Geometry: final body of the model. Coordinates: model frame, mm. Give positions to 0.01 mm unless a question says otherwise; leave off trailing zeros. Write each loop counter-clockwise with the first axis right and the second up, starting at its lowest first coordinate (ties: lowest second). Pieces come first, ordered by that corner, then holes.
Q1. Section B-B (x = -337). Return the cut outline in (y, z) (3 decimals), plus the area to 3 significant figures.
Q2. Section A-A (z = 12.75). Return the cut outline in (x, y), plus the area to 3 significant figures.
Q3. Line query: line 1 (Y direction, x = -16, z = 18); line 2 (X direction, y = 50, z = 16.5); line 3 (X direction, y = 34, z = 8.5). Output: solid intervals per line, ascending.
Q4. Pin query (flat end, axial travel): pin 1 Ø3 at (y, z) = (65, 12) entering from +X; pin 2 Ø1 at (y, z) = (27, 12) entering from -X; pin 3 Ø1 at (y, z) = (34.5, 13) entering from -X. Return the tip coordinate at first contact, or that it passes through.
Q5. Section C-C (y = 15.5). Return the cut outline in (x, z), plus the area to 3 significant figures.
Autodesk Inventor part; units mm, degrees
ref_plane "YZ Plane" through (0, 0, 0) normal (1, 0, 0) x (0, 1, 0)
ref_plane "XZ Plane" through (0, 0, 0) normal (0, 1, 0) x (-1, 0, 0)
ref_plane "XY Plane" through (0, 0, 0) normal (0, 0, 1) x (1, 0, 0)
sketch "Sketch2" plane through (0, 0, 0) normal (0, 0, 1) x (1, 0, 0)
  line L0 (-410.0497, 90.9112) -> (409.1003, 90.9112)
  line L1 (409.1003, 90.9112) -> (409.1003, -10.6888)
  line L2 (409.1003, -10.6888) -> (-410.0497, -10.6888)
  line L3 (-410.0497, -10.6888) -> (-410.0497, 90.9112)
  point P0 (0, 0)
  dimension "d0" = 819.15
  dimension "d1" = 101.6
extrude "Board" add sketch "Sketch2" along normal blind 19.05
sketch "Sketch10" plane through (0, 0, 19.05) normal (0, 0, 1) x (1, 0, 0)
  line L0 (409.1003, -10.6888) -> (409.1003, 90.9112)
  line L1 (409.1003, 81.3862) -> (-410.0497, 81.3862)
  line L2 (-410.0497, 81.3862) -> (-410.0497, 71.8612)
  line L3 (-410.0497, 71.8612) -> (409.1003, 71.8612)
  line L4 (409.1003, 71.8612) -> (409.1003, 81.3862)
  line L5 (-410.0497, 90.9112) -> (-410.0497, -10.6888)
  line L6 (409.1003, 90.9112) -> (-410.0497, 90.9112)
  point P0 (0, 0)
  dimension "d22" = 9.525
  dimension "d23" = 9.525
sketch "Sketch8" plane through (-410.0497, -10.6888, 0) normal (0, -1, 0) x (1, 0, 0)
  line L0 (819.15, 19.05) -> (0, 19.05)
  line L1 (0, 0) -> (0, 19.05)
  line L2 (0, 19.05) -> (0, 0)
  line L3 (0, 0) -> (19.05, 19.05)
  line L4 (19.05, 19.05) -> (0, 19.05)
  line L5 (819.15, 0) -> (819.15, 19.05)
  line L6 (819.15, 19.05) -> (819.15, 0)
  line L7 (819.15, 0) -> (800.1, 19.05)
  line L8 (800.1, 19.05) -> (819.15, 19.05)
  point P0 (410.0497, 0)
  dimension "d15" = 45
  dimension "d16" = 45
extrude "45 degree mitre" cut sketch "Sketch8" against normal blind 101.6
extrude "Extrusion7" cut sketch "Sketch10" against normal blind 9.525 contours L3 L2 L1 L0
equation "\"d17\" = d1"
properties part number "Base Runner Rear"
Computed:
1. outline: (-10.689, 0) - (90.911, 0) - (90.911, 19.05) - (81.386, 19.05) - (81.386, 9.525) - (71.861, 9.525) - (71.861, 19.05) - (-10.689, 19.05) - close
1. area: 1,840 mm2
2. outline: (-397.3, -10.69) - (396.35, -10.69) - (396.35, 71.86) - (-397.3, 71.86) - close; (-397.3, 81.39) - (396.35, 81.39) - (396.35, 90.91) - (-397.3, 90.91) - close
2. area: 73,100 mm2
3. line 1: y = -10.69 to 71.86, 81.39 to 90.91
3. line 2: x = -393.55 to 392.6
3. line 3: x = -401.55 to 400.6
4. pin 1: stops at x = 398.6
4. pin 2: stops at x = -398.55
4. pin 3: stops at x = -397.55
5. outline: (-410.05, 0) - (409.1, 0) - (390.05, 19.05) - (-391, 19.05) - close
5. area: 15,200 mm2
